Read the model definition and answer for the solid it produces. Units are mm, in the model's axes. A direction names the side the tool comes from. Round coordinates to 2 decimals unless told otherwise and drop trailing zeros. Write each loop counter-clockwise with the first axis right and the second up, starting at its lowest first coordinate (ties: lowest second). Pieces come first, ordered by that corner, then holes. Notation, with made-up numbers: (-2.75, 17.25) - (8.25, 17.25) arc R22 cw to (8.25, 36.25) - close; hole circle Ø10 at (19.25, -0.5). An arc over 180 degrees is marked (long way). Use one line per item in the form item = value. Start each with the question number.
1) Consider line 1 along Z through (x, y) = (-28, 10); line 2 along X through (y, z) = (-15, 7); line 3 along X through (y, z) = (-6, 7.5). Determine where each line is inside the solid, lowest interval first. Write a range as from..to.
2) Each of these flat-tipped pins is pushed along its axis until it touches: pin 1 (4 mm diameter, centred on y = -17.5, z = 16, fed in from +X); pin 2 (4 mm diameter, centred on x = 10.5, y = -21, fed in from +Z); pin 3 (2 mm diameter, centred on x = 11, z = 24, fed in from -Y). Where does it stop, or does it pass through?
3) For a pull along X with two mould halves and no side action, classify faces 1 (the face through (-20, 25.4, 12)), 2 (the face through (20.32, 18, 19)), 3 (the face through (-30.48, -11, 19)), 4 (the face through (-25.4, -19, 18)) as released by +X, released by -X, zero draft, split by the parting line, or undercut.
4) The part is cut by section C-C, the plane z = 23. Give the vertices of the cut face in (x, y), plus the area to 3 significant figures.
5) For faces 5 (the face through (-20.32, 18, 19)), 6 (the face through (30.48, -11, 19)), 7 (the face through (0, -12.7, 18)), determine the directions among +Z, -Z, +X, -X, +Y, -Y from which every point of the face is accessible in a straight line to the end or side of a thin tool.
6) The part is cut by section B-B, the plane y = -15. Give the vertices of the cut face in (x, z).
7) The part is cut by section A-A, the plane z = 4. Give the vertices of the cut face in (x, y).
8) The part is cut by section D-D, the plane y = -3.5. Give the vertices of the cut face in (x, z).
from build123d import *

# Parameters (mm, degrees)
F0_W     = 76.2
F0_H     = 50.8
F1_DEPTH = 6.35
F3_DEPTH = 25.4
F5_DEPTH = 31.75
F6_SIZE  = 1.27
F7_R     = 10.16
F8_SIZE  = 1.27
F9_R     = 7.62
F10_R    = 7.62


with BuildPart() as f1:
    # F0 (on Top) → F1 (new body)
    with BuildSketch(Plane.XY):
        Rectangle(F0_W, F0_H)
    extrude(amount=F1_DEPTH)

    # F2 (on face) → F3 (join)
    with BuildSketch(Plane.XY.offset(6.35)):
        Polygon((-25.4, -25.4), (-25.4, -12.7), (-25.4, 3.18004773), (-30.48, 3.18004773), (-30.48, -25.4), align=None)
        Polygon((30.48, 3.18004773), (25.4, 3.18004773), (25.4, -12.7), (25.4, -25.4), (30.48, -25.4), align=None)
        with BuildLine():
            Line((20.32, 3.18004773), (20.32, 25.4))
            Line((20.32, 25.4), (14.478, 25.4))
            ThreePointArc((14.478, 25.4), (-0.9019215927, 10.0200784073), (-16.2818431854, 25.4))
            Line((-16.2818431854, 25.4), (-20.32, 25.4))
            Line((-20.32, 25.4), (-20.32, 3.18004773))
            Line((-20.32, 3.18004773), (-25.4, 3.18004773))
            Line((-25.4, 3.18004773), (-25.4, -12.7))
            Line((-25.4, -12.7), (25.4, -12.7))
            Line((25.4, -12.7), (25.4, 3.18004773))
            Line((25.4, 3.18004773), (20.32, 3.18004773))
        make_face()
    extrude(amount=F3_DEPTH)

    # F4 (on face) → F5 (cut)
    with BuildSketch(Plane.XY.offset(31.75)):
        with BuildLine():
            Line((14.478, 25.4), (-16.2818431854, 25.4))
            ThreePointArc((-16.2818431854, 25.4), (-0.9019215927, 10.0200784073), (14.478, 25.4))
        make_face()
    extrude(amount=-F5_DEPTH, mode=Mode.SUBTRACT)

    # F6
    f6_edges = [f1.edges().sort_by_distance(p)[0] for p in [
        (0, -12.7, 31.75),
        (-25.4, -19.05, 31.75),
        (25.4, -19.05, 31.75),
    ]]
    chamfer(f6_edges, length=F6_SIZE)

    # F7
    f7_edges = [f1.edges().sort_by_distance(p)[0] for p in [
        (-38.1, 25.4, 3.175),
        (38.1, 25.4, 3.175),
    ]]
    fillet(f7_edges, radius=F7_R)

    # F8
    f8_edges = [f1.edges().sort_by_distance(p)[0] for p in [
        (-0.901922, 10.020078, 31.75),
    ]]
    chamfer(f8_edges, length=F8_SIZE)

    # F9
    f9_edges = [f1.edges().sort_by_distance(p)[0] for p in [
        (-20.32, 3.180048, 19.05),
    ]]
    fillet(f9_edges, radius=F9_R)

    # F10
    f10_edges = [f1.edges().sort_by_distance(p)[0] for p in [
        (20.32, 3.180048, 19.05),
    ]]
    fillet(f10_edges, radius=F10_R)


solid = f1.part
Geometry results:
q1.line_1 = 0..6.35
q1.line_2 = -30.48..-25.4, 25.4..30.48
q1.line_3 = -30.48..30.48
q2.pin_1 = 30.48
q2.pin_2 = 6.35
q2.pin_3 = -12.7
q3.face_1 = zero draft
q3.face_2 = released by +X
q3.face_3 = released by -X
q3.face_4 = undercut
q4.outline = (-30.48, -25.4) - (-25.4, -25.4) - (-25.4, -12.7) - (25.4, -12.7) - (25.4, -25.4) - (30.48, -25.4) - (30.48, 3.18) - (27.94, 3.18) arc R7.62 cw to (20.32, 10.8) - (20.32, 25.4) - (14.48, 25.4) arc R15.38 cw to (-16.28, 25.4) - (-20.32, 25.4) - (-20.32, 10.8) arc R7.62 cw to (-27.94, 3.18) - (-30.48, 3.18) - close
q4.area = 1,650 mm2
q5.face_5 = +Z, -X, +Y
q5.face_6 = +Z, +X, +Y, -Y
q5.face_7 = +Z, -Y
q6.outline = (-38.1, 0) - (38.1, 0) - (38.1, 6.35) - (30.48, 6.35) - (30.48, 31.75) - (26.67, 31.75) - (25.4, 30.48) - (25.4, 6.35) - (-25.4, 6.35) - (-25.4, 30.48) - (-26.67, 31.75) - (-30.48, 31.75) - (-30.48, 6.35) - (-38.1, 6.35) - close
q7.outline = (-38.1, -25.4) - (38.1, -25.4) - (38.1, 15.24) arc R10.16 ccw to (27.94, 25.4) - (14.48, 25.4) arc R15.38 cw to (-16.28, 25.4) - (-27.94, 25.4) arc R10.16 ccw to (-38.1, 15.24) - close
q8.outline = (-38.1, 0) - (38.1, 0) - (38.1, 6.35) - (30.48, 6.35) - (30.48, 31.75) - (-30.48, 31.75) - (-30.48, 6.35) - (-38.1, 6.35) - close
